from build123d import *

# Parameters (mm, degrees)
SKETCH1_W             = 24.8
SKETCH1_H             = 25.8
BOSS_EXTRUDE1_DEPTH   = 1
SKETCH3_W             = 16.2
SKETCH3_H             = 7
BOSS_EXTRUDE3_DEPTH   = 17.8
DRAFT2_ANGLE          = 45
TOP_FILLET_R          = 5
SKETCH4_R             = 2.65
HOLE_BOLT_DEPTH       = 4
SKETCH5_R             = 4.5
HOLE_BOLT_CAP_DEPTH   = 20
SKETCH6_R             = 1.2
HOLES_DOWEL_PIN_DEPTH = 2.5
BASE_FILLET_R         = 3
BRIM_DEPTH            = 0.65
INWARD_SLANT_ANGLE    = 2.5
FILLET1_START         = 8.48845
FILLET1_2_DEPTH       = 24.8
FILLET1_3_DEPTH       = 1.3
FILLET1_START_2       = 31.98845
FILLET1_4_DEPTH       = 1.3
FILLET1_START_3       = -20
FILLET1_5_DEPTH       = 28


with BuildPart() as part:
    # Sketch1 → Boss-Extrude1 (new body)
    with BuildSketch(Plane(origin=(0, 0, 0), x_dir=(1, 0, 0), z_dir=(0, 1, 0))):
        with Locations((20.88845, 5.671213532)):
            Rectangle(SKETCH1_W, SKETCH1_H)
    extrude(amount=BOSS_EXTRUDE1_DEPTH)

    # Sketch3 → Boss-Extrude3 (add)
    with BuildSketch(Plane(origin=(0, 1, 0), x_dir=(1, 0, 0), z_dir=(0, 1, 0))):
        with Locations((20.88845, -3.728786468)):
            Rectangle(SKETCH3_W, SKETCH3_H)
    extrude(amount=BOSS_EXTRUDE3_DEPTH)

    # Draft2
    draft2_faces = [part.faces().sort_by_distance(p)[0] for p in [
        (20.88845, 9.9, 0.228786468),
    ]]
    draft(draft2_faces, Plane.ZX.offset(18.8), DRAFT2_ANGLE)

    # top_fillet
    top_fillet_edges = [part.edges().sort_by_distance(p)[0] for p in [
        (12.78845, 18.8, 3.728786468),
        (28.98845, 18.8, 3.728786468),
    ]]
    fillet(top_fillet_edges, radius=TOP_FILLET_R)

    # Sketch4 → hole_bolt (cut)
    with BuildSketch(Plane.XY.offset(7.228786468)):
        with Locations((20.88845, 13.5)):
            Circle(SKETCH4_R)
    extrude(amount=-HOLE_BOLT_DEPTH, mode=Mode.SUBTRACT)

    # Sketch5 → hole_bolt_cap (cut)
    with BuildSketch(Plane.XY.offset(3.228786468)):
        with Locations((20.88845, 13.5)):
            Circle(SKETCH5_R)
    extrude(amount=-HOLE_BOLT_CAP_DEPTH, mode=Mode.SUBTRACT)

    # Sketch6 → holes_dowel_pin (cut)
    with BuildSketch(Plane.XY.offset(7.228786468)):
        with Locations((25.38845, 13.5)):
            Circle(SKETCH6_R)
        with Locations((16.38845, 13.5)):
            Circle(SKETCH6_R)
    extrude(amount=-HOLES_DOWEL_PIN_DEPTH, mode=Mode.SUBTRACT)

    # base_fillet
    # the kernel refuses this fillet: 3 mm, written as the material it adds along each edge
    with BuildSketch(Plane(origin=(12.78845, 1, -25.071213532), x_dir=(-1, 0, 0), z_dir=(0, 0, 1))) as base_fillet_piece_1_section:
        with BuildLine():
            CenterArc((BASE_FILLET_R, -BASE_FILLET_R), BASE_FILLET_R, 90, 90)
            Line((0, -BASE_FILLET_R), (0, 0))
            Line((0, 0), (BASE_FILLET_R, 0))
        make_face()
    base_fillet_piece_1 = extrude(amount=32.3, mode=Mode.PRIVATE)
    base_fillet_piece_1 = split(base_fillet_piece_1, bisect_by=Plane(origin=(12.78845, -2.75, -21.321213532), z_dir=(0, -0.7071067811865488, 0.7071067811865462)), keep=Keep.TOP, mode=Mode.PRIVATE)
    add(base_fillet_piece_1)
    with BuildSketch(Plane(origin=(28.98845, 1, 7.228786468), x_dir=(0, 1, 0), z_dir=(0, 0, -1))) as base_fillet_piece_2_section:
        with BuildLine():
            CenterArc((BASE_FILLET_R, BASE_FILLET_R), BASE_FILLET_R, 180, 90)
            Line((0, BASE_FILLET_R), (0, 0))
            Line((0, 0), (BASE_FILLET_R, 0))
        make_face()
    base_fillet_piece_2 = extrude(amount=32.3, mode=Mode.PRIVATE)
    base_fillet_piece_2 = split(base_fillet_piece_2, bisect_by=Plane(origin=(28.98845, 13.4, -5.171213532), z_dir=(0, -0.7071067811865488, 0.7071067811865462)), keep=Keep.TOP, mode=Mode.PRIVATE)
    add(base_fillet_piece_2)
    with BuildSketch(Plane(origin=(28.98845, 1, -17.571213532), x_dir=(0, 0, -1), z_dir=(-1, 0, 0))) as base_fillet_piece_3:
        with BuildLine():
            CenterArc((1.25335823, -2.989282457), BASE_FILLET_R, 94.844556223, 40.155443777)
            Line((-0.867962113, -0.867962113), (0, 0))
            Line((0, 0), (1, 0))
        make_face()
    extrude(amount=16.2)
    with BuildSketch(Plane(origin=(12.78845, 1, -25.071213532), x_dir=(-1, 0, 0), z_dir=(0, 0, 1))) as base_fillet_piece_4a_section:
        with BuildLine():
            CenterArc((BASE_FILLET_R, -BASE_FILLET_R), BASE_FILLET_R, 90, 90)
            Line((0, -BASE_FILLET_R), (0, 0))
            Line((0, 0), (BASE_FILLET_R, 0))
        make_face()
    base_fillet_piece_4a = extrude(amount=32.3, mode=Mode.PRIVATE)
    base_fillet_piece_4a = split(base_fillet_piece_4a, bisect_by=Plane(origin=(12.78845, -2.75, -21.321213532), z_dir=(0, 0.7071067811865488, -0.7071067811865462)), keep=Keep.TOP, mode=Mode.PRIVATE)
    base_fillet_piece_4a = split(base_fillet_piece_4a, bisect_by=Plane(origin=(12.78845, 1, -18.571213532), z_dir=(0, 0, 1)), keep=Keep.TOP, mode=Mode.PRIVATE)
    with BuildSketch(Plane(origin=(28.98845, 1, -17.571213532), x_dir=(0, 0, -1), z_dir=(-1, 0, 0))) as base_fillet_piece_4b_section:
        with BuildLine():
            CenterArc((1.25335823, -2.989282457), BASE_FILLET_R, 94.844556223, 40.155443777)
            Line((-0.867962113, -0.867962113), (0, 0))
            Line((0, 0), (1, 0))
        make_face()
    base_fillet_piece_4b = extrude(amount=19.268709481, mode=Mode.PRIVATE)
    base_fillet_piece_4b = split(base_fillet_piece_4b, bisect_by=Plane(origin=(12.78845, 1, -17.571213532), z_dir=(-1, 0, 0)), keep=Keep.TOP, mode=Mode.PRIVATE)
    base_fillet_piece_4 = base_fillet_piece_4a & base_fillet_piece_4b
    add(base_fillet_piece_4)
    with BuildSketch(Plane(origin=(28.98845, 1, 7.228786468), x_dir=(0, 1, 0), z_dir=(0, 0, -1))) as base_fillet_piece_5a_section:
        with BuildLine():
            CenterArc((BASE_FILLET_R, BASE_FILLET_R), BASE_FILLET_R, 180, 90)
            Line((0, BASE_FILLET_R), (0, 0))
            Line((0, 0), (BASE_FILLET_R, 0))
        make_face()
    base_fillet_piece_5a = extrude(amount=32.3, mode=Mode.PRIVATE)
    base_fillet_piece_5a = split(base_fillet_piece_5a, bisect_by=Plane(origin=(28.98845, 13.4, -5.171213532), z_dir=(0, 0.7071067811865488, -0.7071067811865462)), keep=Keep.TOP, mode=Mode.PRIVATE)
    base_fillet_piece_5a = split(base_fillet_piece_5a, bisect_by=Plane(origin=(28.98845, 1, -18.571213532), z_dir=(0, 0, 1)), keep=Keep.TOP, mode=Mode.PRIVATE)
    with BuildSketch(Plane(origin=(32.057159481, 1, -17.571213532), x_dir=(0, 0, -1), z_dir=(-1, 0, 0))) as base_fillet_piece_5b_section:
        with BuildLine():
            CenterArc((1.25335823, -2.989282457), BASE_FILLET_R, 94.844556223, 40.155443777)
            Line((-0.867962113, -0.867962113), (0, 0))
            Line((0, 0), (1, 0))
        make_face()
    base_fillet_piece_5b = extrude(amount=19.268709481, mode=Mode.PRIVATE)
    base_fillet_piece_5b = split(base_fillet_piece_5b, bisect_by=Plane(origin=(28.98845, 1, -17.571213532), z_dir=(1, 0, 0)), keep=Keep.TOP, mode=Mode.PRIVATE)
    base_fillet_piece_5 = base_fillet_piece_5a & base_fillet_piece_5b
    add(base_fillet_piece_5)

    # Sketch8 → brim (add)
    with BuildSketch(Plane.XZ):
        Polygon((8.48845, 7.228786468), (9.58845, 7.228786468), (9.58845, -17.471213532), (32.18845, -17.471213532), (32.18845, 7.228786468), (33.28845, 7.228786468), (33.28845, -18.571213532), (8.48845, -18.571213532), align=None)
    extrude(amount=BRIM_DEPTH)

    # inward_slant
    inward_slant_faces = [part.faces().sort_by_distance(p)[0] for p in [
        (20.88845, 8.182651501, 7.228786468),
    ]]
    draft(inward_slant_faces, Plane(origin=(0, 0, 0), x_dir=(0, 0, -1), z_dir=(0, -1, 0)), INWARD_SLANT_ANGLE)

    # Fillet1: read off the stored shape, not the designer's step
    # Fillet1 outline → Fillet1 (revolve, cut)
    with BuildSketch(Plane(origin=(9.78845, 4, 0), x_dir=(1, 0, 0), z_dir=(0, -1, 0))):
        with BuildLine():
            ThreePointArc((4, -18.571213532), (3.292893219, -18.278320313), (3, -17.571213532))
            Line((3, -17.571213532), (3, -18.571213532))
            Line((3, -18.571213532), (4, -18.571213532))
        make_face()
    revolve(axis=Axis((9.78845, 4, 0), (0, 0, 1)), mode=Mode.SUBTRACT)

    # Fillet1 2 outline → Fillet1 2 (cut)
    with BuildSketch(Plane.YZ.offset(FILLET1_START)):
        with BuildLine():
            Line((1, -18.254186707), (1, -18.158633642))
            ThreePointArc((1, -18.158633642), (0.644909369, -18.462117598), (0.19071784, -18.571213532))
            Line((0.19071784, -18.571213532), (1, -18.571213532))
            Line((1, -18.571213532), (1, -18.254186707))
        make_face()
        with BuildLine():
            ThreePointArc((1.140358994, -17.884553089), (1.080792468, -18.027028359), (1, -18.158633642))
            Line((1, -18.158633642), (1, -18.254186707))
            Line((1, -18.254186707), (0.999995093, -18.571271439))
            ThreePointArc((0.999995093, -18.571271439), (1.050052637, -18.223798874), (1.140358994, -17.884553089))
        make_face()
    extrude(amount=FILLET1_2_DEPTH, mode=Mode.SUBTRACT)

    # Fillet1 3 outline → Fillet1 3 (cut)
    with BuildSketch(Plane.YZ.offset(FILLET1_START)):
        with BuildLine():
            Line((1, -18.158633642), (1, -17.571213532))
            ThreePointArc((1, -17.571213532), (0.707106781, -18.278320313), (0, -18.571213532))
            Line((0, -18.571213532), (0.19071784, -18.571213532))
            ThreePointArc((0.19071784, -18.571213532), (0.644909369, -18.462117598), (1, -18.158633642))
        make_face()
    extrude(amount=FILLET1_3_DEPTH, mode=Mode.SUBTRACT)

    # Fillet1 4 outline → Fillet1 4 (cut)
    with BuildSketch(Plane.YZ.offset(FILLET1_START_2)):
        with BuildLine():
            Line((1, -18.158633642), (1, -17.571213532))
            ThreePointArc((1, -17.571213532), (0.707106781, -18.278320313), (0, -18.571213532))
            Line((0, -18.571213532), (0.19071784, -18.571213532))
            ThreePointArc((0.19071784, -18.571213532), (0.644909369, -18.462117598), (1, -18.158633642))
        make_face()
    extrude(amount=FILLET1_4_DEPTH, mode=Mode.SUBTRACT)

    # Fillet1 5 outline → Fillet1 5 (cut)
    with BuildSketch(Plane.XY.offset(FILLET1_START_3)):
        with BuildLine():
            ThreePointArc((8.48845, 0), (8.781343219, 0.707106781), (9.48845, 1))
            Line((9.48845, 1), (8.48845, 1))
            Line((8.48845, 1), (8.48845, 0))
        make_face()
        with BuildLine():
            Line((33.28845, 1), (32.28845, 1))
            ThreePointArc((32.28845, 1), (32.995556781, 0.707106781), (33.28845, 0))
            Line((33.28845, 0), (33.28845, 1))
        make_face()
    extrude(amount=FILLET1_5_DEPTH, mode=Mode.SUBTRACT)

    # Fillet1 6 outline → Fillet1 6 (revolve, cut)
    with BuildSketch(Plane(origin=(31.98845, 4, 0), x_dir=(1, 0, 0), z_dir=(0, -1, 0))):
        with BuildLine():
            ThreePointArc((4, -18.571213532), (3.292893219, -18.278320313), (3, -17.571213532))
            Line((3, -17.571213532), (3, -18.571213532))
            Line((3, -18.571213532), (4, -18.571213532))
        make_face()
    revolve(axis=Axis((31.98845, 4, 0), (0, 0, 1)), mode=Mode.SUBTRACT)


solid = part.part
Build history of the part. All positions in model axes, mm. A direction names the side the tool comes from. Round coordinates to 2 decimals unless told otherwise and drop trailing zeros. Write each loop counter-clockwise with the first axis right and the second up, starting at its lowest first coordinate (ties: lowest second). Pieces come first, ordered by that corner, then holes. Notation, with made-up numbers: M -10,21.5 L 24,21.5 A31 cw 24,50.5 Z; hole C 84,2.5 d11. An arc over 180 degrees is marked long. Answer as a JSON object with one key per item and string values. Group by question number.
(1) Mould opens along X. For faces 5 (the cylindrical face through (15.436, 12.77, 6.327)), 6 (the flat face through (20.715, 7.05, 7.537)), 7 (the cylindrical face through (19.913, 9.107, -1.659)), 8 (the cylindrical face through (33, 0.7, -5.8)) say: pulls with the +X half, pulls with the -X half, needs draft (parallel to the pull), parting line crosses it, or undercut.
(2) Cut at B-B (x = 27.75). Give the cut face in (y, z), and give its area (3 significant figures).
(3) Cut at C-C (z = -11). Give the cut face in (x, y), and give its area (3 significant figures).
(4) Which spindle directions (+Z, -Z, +X, -X, +Y, -Y) get a long thin tool onto all of the face, cutting with end or side? Do faces 1 (the flat face through (24, 14, 3.229)), 2 (the flat face through (16, 14, 4.729)), 3 (the flat face through (28.988, 9, -1)), 4 (the flat face through (21, 0, -5)). Say none if no direction does.
(5) Flat gauge pins, fed straight in: pin 1 (2 mm diameter, centred on x = 21.5, z = -1, fed in from +Y); pin 2 (8 mm diameter, centred on y = 13.5, z = 3.5, fed in from -X); pin 3 (5.5 mm diameter, centred on x = 20.89, y = 13.5, fed in from +Z); pin 4 (5 mm diameter, centred on x = 20.89, y = 13.5, fed in from +Z) (1 decimal). Where does each tip first touch, or does it go through?
(6) Cut at A-A (y = 11.25). Give the cut face in (x, z), and give its area (3 significant figures).
(7) Cut at D-D (y = 15.5). Give the cut face in (x, z).
(8) Drill centre lines: L1, parallel to X at y = 13.5, z = 6.15; L2, parallel to Y at x = 30.75, z = -1; L3, parallel to X at y = 4, z = 0.5. Where is each one in solid material? Low to high.
Responses:
{
 "1": {"face 5": "undercut", "face 6": "needs draft", "face 7": "undercut", "face 8": "pulls with the +X half"},
 "2": {"outline": "M -0.65,-18.57 L 0.19,-18.57 A1 ccw 1.14,-17.88 A3 cw 1.87,-16.7 L 17.09,-1.48 L 17.09,7.98 L 0,7.23 L 0,-17.47 L -0.65,-17.47 Z", "area": "303 mm2"},
 "3": {"outline": "M 8.49,-0.65 L 9.59,-0.65 L 9.59,0 L 32.19,0 L 32.19,-0.65 L 33.29,-0.65 L 33.29,0 A1 ccw 32.29,1 L 31.99,1 A3 cw 28.99,4 L 28.99,7.57 L 12.79,7.57 L 12.79,4 A3 cw 9.79,1 L 9.49,1 A1 ccw 8.49,0 Z", "area": "136 mm2"},
 "4": {"face 1": "-Z", "face 2": "+Z", "face 3": "+Z, -Z, +X, +Y", "face 4": "+Z, -Y"},
 "5": {"pin 1": "stops at y = 18.57", "pin 2": "stops at x = 12.79", "pin 3": "stops at z = 7.94", "pin 4": "passes through"},
 "6": {"outline": "M 12.79,-7.32 L 16.99,-7.32 L 16.99,3.23 L 19.49,3.23 L 19.49,7.72 L 12.79,7.72 Z; M 22.29,3.23 L 24.79,3.23 L 24.79,-7.32 L 28.99,-7.32 L 28.99,7.72 L 22.29,7.72 Z", "area": "149 mm2"},
 "7": {"outline": "M 13.09,-3.07 L 16.86,-3.07 L 16.86,3.23 L 19.15,3.23 L 19.15,7.91 L 13.09,7.91 Z; M 22.63,3.23 L 24.92,3.23 L 24.92,-3.07 L 28.69,-3.07 L 28.69,7.91 L 22.63,7.91 Z"},
 "8": {"L1": "x = 12.79 to 15.19, 17.59 to 18.24, 23.54 to 24.19, 26.59 to 28.99", "L2": "y = 0 to 1.27", "L3": "x = 12.79 to 28.99"}
}
